Can you work these out from the model? Positions are in its coordinate system, mm. Face numbers are marked on the shaded views. Give positions to 0.01 mm unless a question says otherwise; leave off trailing zeros. Write each loop counter-clockwise with the first axis right and the second up, starting at its lowest first coordinate (ties: lowest second). Pieces come first, ordered by that corner, then holes.
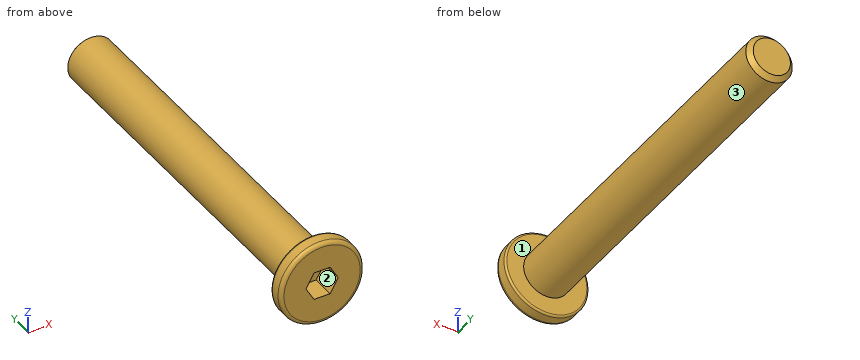
Autodesk Inventor part; units mm, degrees
ref_plane "YZ Plane" through (0, 0, 0) normal (1, 0, 0) x (0, 1, 0)
ref_plane "XZ Plane" through (0, 0, 0) normal (0, 1, 0) x (-1, 0, 0)
ref_plane "XY Plane" through (0, 0, 0) normal (0, 0, 1) x (1, 0, 0)
sketch "Boceto1" plane through (0, 0, 0) normal (0, 1, 0) x (-1, 0, 0)
  circle A0 centre (0, 0) radius 4.5
  dimension "d0" = 9
extrude "Extrusión1" add sketch "Boceto1" along normal blind 1.6
sketch "Boceto2" plane through (0, 1.6, 0) normal (0, 1, 0) x (1, 0, 0)
  circle A0 centre (0, 0) radius 2.5
  dimension "d3" = 5
extrude "Extrusión2" add sketch "Boceto2" along normal blind 40
fillet "Empalme1" radius 0.4 1 edges at (4.5, 0, 0)
fillet "Empalme2" radius 0.2 1 edges at (4.5, 1.6, 0)
sketch "Boceto3" plane through (0, 0, 0) normal (0, -1, 0) x (1, 0, 0)
  line L0 (-1.7321, 0) -> (-0.866, 1.5)
  line L1 (-0.866, 1.5) -> (0.866, 1.5)
  line L2 (0.866, 1.5) -> (1.7321, 0)
  line L3 (1.7321, 0) -> (0.866, -1.5)
  line L4 (0.866, -1.5) -> (-0.866, -1.5)
  line L5 (-0.866, -1.5) -> (-1.7321, 0)
  point P0 (0, 0)
  point P1 (0, 0)
  dimension "d8" = 3
extrude "Extrusión3" cut sketch "Boceto3" against normal blind 2.5
chamfer "Chaflán1" distance 0.5 angle 45 1 edges at (-2.5, 41.6, 0)
thread "Rosca2"
properties part number "Perno M5x8cabeza plana_" material "Hierro, gris"
1) Please list where these lines run through material, in increasing order: L1, parallel to Y at x = 1, z = 1; L2, parallel to Y at x = -1.75, z = -3.25; L3, parallel to Z at x = 0, y = 23.
Values follow:
L1: y = 2.5 to 41.6
L2: y = 0 to 1.6
L3: z = -2.5 to 2.5
2) For pin 1 Ø5 at (y, z) = (5, -2) entering from -X; pin 2 Ø4 at (y, z) = (15.5, 2) entering from +X; pin 3 Ø0.5 at (x, y) = (-0.5, 1) entering from +Z, each with a flat end and sliding along its axis, tell me the tip position at first contact or that it passes through.
Values follow:
pin 1: stops at x = -2.5
pin 2: stops at x = 2.5
pin 3: stops at z = 4.49
3) Suppose I cut it at A-A on x = 0. Write out the boundary of the cut face in (y, z).
Values follow:
outline: (0, -4.1) arc R0.4 ccw to (0.4, -4.5) - (1.4, -4.5) arc R0.2 ccw to (1.6, -4.3) - (1.6, -2.5) - (41.1, -2.5) - (41.6, -2) - (41.6, 2) - (41.1, 2.5) - (1.6, 2.5) - (1.6, 4.3) arc R0.2 ccw to (1.4, 4.5) - (0.4, 4.5) arc R0.4 ccw to (0, 4.1) - (0, 1.5) - (2.5, 1.5) - (2.5, -1.5) - (0, -1.5) - close
4) If we mould it in two halves opening along X, with no side actions, what happens to the marked faces 1, 2 and 3? For each: +X half, -X half, draft (parallel to the pull), parting line (faces both ways), or undercut.
Values follow:
face 1: draft
face 2: undercut
face 3: parting line
5) Suppose I cut it at B-B on y = 35.5. Write out the boundary of the cut face in (x, z).
Values follow:
outline: circle Ø5 at (0, 0)
